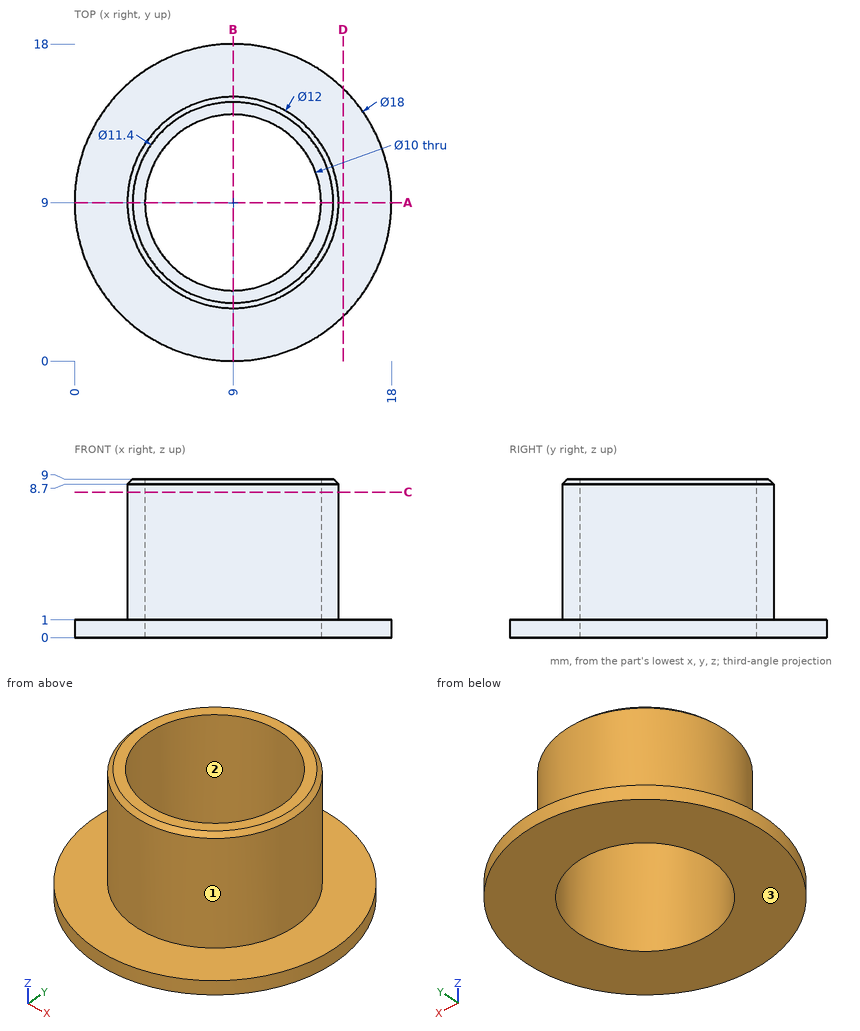
For this review, use the dimensioned drawing (mm, ordinates from the lowest corner) and the shaded views. Round coordinates to 2 decimals unless told otherwise and drop trailing zeros. Order: outer loops, then holes, each group sorted by start corner. A loop starts at its lowest first (then second) coordinate and runs counter-clockwise, first axis right, second up. Notation, with made-up numbers: (4, 11.25) -> (12, 11.25) arc R29 ccw to (12, 35.25) -> close; hole circle Ø1 at (67.25, -37.75). An arc over 180 degrees is marked (long way). Write item = value, one per line. Start each with the question number.
Item 1: Consider section D-D on x = 15.25. Write out the cut boundary in (y, z), plus the area to 3 significant figures.
Item 2: For line 1 along Y through (x, z) = (9, 6.25); line 2 along Z through (x, y) = (12.5, 17.25); line 3 along X through (y, z) = (13, 5.25), list the stretches that pass through material, from the lowest coordinate up.
Item 3: Consider section A-A on y = 9. Write out the cut boundary in (x, z), plus the area to 3 significant figures.
Item 4: Mouldability with a two-part tool opening along X and no side actions: class the marked faces 1, 2 and 3 as released by +X, released by -X, zero draft, split by the parting line, or undercut.
Item 5: Consider section C-C on z = 8.25. Write out the cut boundary in (x, y), plus the area to 3 significant figures.
Item 6: Clearance check with flat-ended pins moving along their axes: pin 1 Ø4 at (y, z) = (12, 6.5) entering from +X; pin 2 Ø4 at (y, z) = (12, 4.5) entering from -X; pin 3 Ø2 at (y, z) = (13, 4.5) entering from -X; pin 4 Ø2 at (x, y) = (12, 12) entering from -Z. State where each tip first meets the part, or that it passes through.
Conclusion:
q1.outline = (2.52, 0) -> (15.48, 0) -> (15.48, 1) -> (2.52, 1) -> close
q1.area = 13.0 mm2
q2.line_1 = 3 to 4, 14 to 15
q2.line_2 = 0 to 1
q2.line_3 = 4.53 to 6, 12 to 13.47
q3.outline = (0, 0) -> (4, 0) -> (4, 9) -> (3.3, 9) -> (3, 8.7) -> (3, 1) -> (0, 1) -> close; (14, 0) -> (18, 0) -> (18, 1) -> (15, 1) -> (15, 8.7) -> (14.7, 9) -> (14, 9) -> close
q3.area = 23.9 mm2
q4.face_1 = split by the parting line
q4.face_2 = undercut
q4.face_3 = zero draft
q5.outline = circle Ø12 at (9, 9); hole circle Ø10 at (9, 9)
q5.area = 34.6 mm2
q6.pin_1 = 14.92
q6.pin_2 = 3.08
q6.pin_3 = 3.8
q6.pin_4 = 0
